Geometry check sheet. Reference: the model listing, model coordinates, mm. A direction names the side the tool comes from. Give positions to 0.01 mm unless a question says otherwise; leave off trailing zeros. Write each loop counter-clockwise with the first axis right and the second up, starting at its lowest first coordinate (ties: lowest second). Pieces come first, ordered by that corner, then holes.
(1) Cross-section at B-B (y = 2.35). Record the boundary of the cut face in (x, z).
(2) Cross-section at D-D (x = 20). Record the boundary of the cut face in (y, z), and give its area (3 significant figures).
(3) Tool access check on faces 1 (the flat face through (30, 1.5, -17)), 2 (the flat face through (54, 2, -2)), 3 (the flat face through (17, 2, -1)), 4 (the flat face through (59, 2, -17)). Record the directions out of +Z, -Z, +X, -X, +Y, -Y that give a thin tool (end or side, any length) a straight path to the whole face; none if there is none.
(4) Depth check by flat-ended pin: P1, Ø1.6, axis at x = 18.5, y = 2.5, coming from the -Z side; P2, Ø0.6, axis at x = 24.5, z = -1, coming from the +Y side; P3, Ø0.8, axis at x = 9.5, y = 1, coming from the -Z side. Enter the tip coordinate at first touch or a pass-through.
(5) Cross-section at C-C (z = -9). Record the boundary of the cut face in (x, y).
(6) Thickness scan on line 1 along X through (y, z) = (1.8, -1); line 2 along Z through (x, y) = (32.5, 1.85); line 3 along Y through (x, z) = (41.5, -16.5). Record the ranges inside material, lowest first.
(7) Mould release check, pull along Z, two halves, no side actions. Record for faces 5 (the flat face through (2, 2, -17)), 6 (the flat face through (14, 2, 1)), 7 (the flat face through (49, 1, -34)), 8 (the flat face through (30, 2, -30)): +Z half, -Z half, draft (parallel to the pull), parting line (faces both ways), or undercut.
(8) Cross-section at A-A (x = 30.5). Record the boundary of the cut face in (y, z), and give its area (4 significant figures).
```python
from build123d import *

# Parameters (mm, degrees)
SKETCH1_W             = 61
SKETCH1_H             = 34
BOSS_EXTRUDE1_DEPTH   = 1.5
SKETCH2_W             = 57
SKETCH2_H             = 30
BOSS_EXTRUDE2_DEPTH   = 1.5
SKETCH3_W             = 53
SKETCH3_H             = 26
CUT_EXTRUDE1_DEPTH    = 1.5
SKETCH4_R             = 6
BOSS_EXTRUDE3_DEPTH   = 1.5
M3_TAPPED_HOLE2_D     = 2.5
M3_TAPPED_HOLE2_DEPTH = 7.5
M3_TAPPED_HOLE2_TIP   = 0.751075774
SKETCH9_W             = 5
SKETCH9_H             = 1.5
BOSS_EXTRUDE4_DEPTH   = 3


with BuildPart() as part:
    # Sketch1 → Boss-Extrude1 (new body)
    with BuildSketch(Plane(origin=(0, 0, 0), x_dir=(1, 0, 0), z_dir=(0, 1, 0))):
        with Locations((30.5, 17)):
            Rectangle(SKETCH1_W, SKETCH1_H)
    extrude(amount=BOSS_EXTRUDE1_DEPTH)

    # Sketch2 → Boss-Extrude2 (add)
    with BuildSketch(Plane(origin=(0, 1.5, 0), x_dir=(1, 0, 0), z_dir=(0, 1, 0))):
        with Locations((30.5, 17)):
            Rectangle(SKETCH2_W, SKETCH2_H)
    extrude(amount=BOSS_EXTRUDE2_DEPTH)

    # Sketch3 → Cut-Extrude1 (cut)
    with BuildSketch(Plane(origin=(0, 3, 0), x_dir=(1, 0, 0), z_dir=(0, 1, 0))):
        with Locations((30.5, 17)):
            Rectangle(SKETCH3_W, SKETCH3_H)
    extrude(amount=-CUT_EXTRUDE1_DEPTH, mode=Mode.SUBTRACT)

    # Sketch4 → Boss-Extrude3 (add)
    with BuildSketch(Plane(origin=(0, 0, 0), x_dir=(-1, 0, 0), z_dir=(0, -1, 0))):
        with Locations((-30.5, 34)):
            Circle(SKETCH4_R)
    extrude(amount=-BOSS_EXTRUDE3_DEPTH)

    # M3 Tapped Hole2
    with Locations(Plane(origin=(30.5, 0, -37), x_dir=(0, 0, -1), z_dir=(0, -1, 0))):
        with Locations((0, 0)):
            Hole(M3_TAPPED_HOLE2_D / 2, depth=M3_TAPPED_HOLE2_DEPTH)
            with Locations((0, 0, -(M3_TAPPED_HOLE2_DEPTH + M3_TAPPED_HOLE2_TIP / 2))):  # 118° drill point
                Cone(0, M3_TAPPED_HOLE2_D / 2, M3_TAPPED_HOLE2_TIP, mode=Mode.SUBTRACT)

    # Sketch9 → Boss-Extrude4 (add)
    with BuildSketch(Plane.XY.offset(-2)):
        with Locations((14.5, 2.25)):
            Rectangle(SKETCH9_W, SKETCH9_H)
        with Locations((46.5, 2.25)):
            Rectangle(SKETCH9_W, SKETCH9_H)
    extrude(amount=BOSS_EXTRUDE4_DEPTH)


solid = part.part
```
Reply:
1. outline: (2, -32) - (59, -32) - (59, -2) - (49, -2) - (49, 1) - (44, 1) - (44, -2) - (17, -2) - (17, 1) - (12, 1) - (12, -2) - (2, -2) - close; hole (4, -30) - (57, -30) - (57, -4) - (4, -4) - close
2. outline: (0, -34) - (1.5, -34) - (1.5, -32) - (3, -32) - (3, -30) - (1.5, -30) - (1.5, -4) - (3, -4) - (3, -2) - (1.5, -2) - (1.5, 0) - (0, 0) - close
2. area: 57.0 mm2
3. face 1: +Y
3. face 2: +Z, +X, +Y
3. face 3: +Z, +Y
3. face 4: +Z, -Z, +X, +Y
4. P1: stops at z = -32
4. P2: stops at y = 1.5
4. P3: stops at z = -34
5. outline: (0, 0) - (61, 0) - (61, 1.5) - (59, 1.5) - (59, 3) - (57, 3) - (57, 1.5) - (4, 1.5) - (4, 3) - (2, 3) - (2, 1.5) - (0, 1.5) - close
6. line 1: x = 12 to 17, 44 to 49
6. line 2: z = -32 to -30, -4 to -2
6. line 3: y = 0 to 1.5
7. face 5: draft
7. face 6: +Z half
7. face 7: -Z half
7. face 8: undercut
8. outline: (0, -40) - (1.5, -40) - (1.5, -38.25) - (0, -38.25) - close; (0, -35.75) - (1.5, -35.75) - (1.5, -32) - (3, -32) - (3, -30) - (1.5, -30) - (1.5, -4) - (3, -4) - (3, -2) - (1.5, -2) - (1.5, 0) - (0, 0) - close
8. area: 62.25 mm2
